Design review of the part built by this model. Coordinates are the model's own, in mm. Coordinates: 2 decimals unless noted, no trailing zeros. Answer as a JSON object with one key per item and string values.
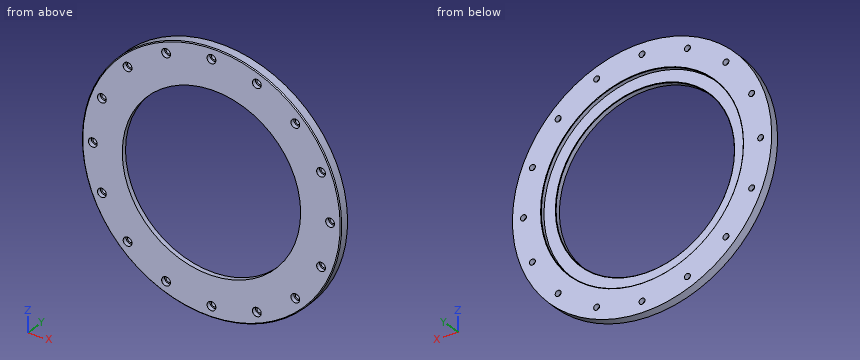
```python
from build123d import *

# Parameters (mm, degrees)
CIRPATTERN1_COUNT = 16
CHAMFER1_SIZE     = 1
CHAMFER2_SIZE     = 2


with BuildPart() as part:
    # Sketch1 → Revolve1 (revolve)
    with BuildSketch(Plane.XY, mode=Mode.PRIVATE) as revolve1_sk:
        Polygon((-203, 0), (-295, 0), (-295, 22), (-230, 22), (-230, 12), (-203, 12), align=None)
    revolve(revolve1_sk.sketch.rotate(Axis((0, 0, 0), (0, 1, 0)), 270), axis=Axis((0, 0, 0), (0, 1, 0)))

    # Sketch4 → CBORE for M12 SHCS1 (revolve, cut)
    with BuildSketch(Plane(origin=(0, 0, 270), x_dir=(0, 0, -1), z_dir=(1, 0, 0))):
        Polygon((0, 0), (0, 22), (6.75, 22), (6.75, 10), (10, 10), (10, 0.025), (10.025, 0), align=None)
    cbore_for_m12_shcs1 = revolve(axis=Axis((0, -6.35, 270), (0, 1, 0)), mode=Mode.SUBTRACT)

    # CirPattern1: CBORE for M12 SHCS1 ×16 about axis
    cirpattern1_axis = Axis((0, 0, 0), (0, 1, 0))
    for i in range(1, CIRPATTERN1_COUNT):
        add(cbore_for_m12_shcs1.rotate(cirpattern1_axis, i * 360 / CIRPATTERN1_COUNT), mode=Mode.SUBTRACT)

    # Chamfer1
    chamfer1_edges = [part.edges().sort_by_distance(p)[0] for p in [
        (0, 12, 203),
        (0, 22, 230),
    ]]
    chamfer(chamfer1_edges, length=CHAMFER1_SIZE)

    # Chamfer2
    chamfer2_edges = [part.edges().sort_by_distance(p)[0] for p in [
        (0, 0, 295),
    ]]
    chamfer(chamfer2_edges, length=CHAMFER2_SIZE)


solid = part.part
```
1) Wall thickness on probe 1 along Z at (x, y) = (-8, 15.5); probe 2 along X at (y, z) = (10.25, -186); probe 3 along Z at (x, y) = (-185, 17.5): over which ranges is each line inside the solid? List them lowest first.
Completed:
{"probe 1": "-294.89 to -229.86, 229.86 to 294.89", "probe 2": "-228.97 to -195.54, -186.3 to -81.32, 81.32 to 186.3, 195.54 to 228.97", "probe 3": "-229.78 to -194.16, -187.67 to -136.66, 136.66 to 187.67, 194.16 to 229.78"}
2) Clearance check with flat-ended pins moving along their axes: pin 1 Ø8 at (y, z) = (10, -186) entering from -X; pin 2 Ø10 at (x, y) = (-123, 17) entering from -Z; pin 3 Ø1.5 at (y, z) = (19.5, -180.5) entering from -X; pin 4 Ø11 at (x, z) = (-190.92, 190.92) entering from +Y. State where each tip first meets the part, or that it passes through.
Completed:
{"pin 1": "x = -232.17", "pin 2": "z = -270.37", "pin 3": "x = -233.91", "pin 4": "through"}
3) Add section A-A, the plane z = 0. Count the separate pieces of the cut face and the enclosed holes in it, and give its area (3 significant figures).
Completed:
{"separate pieces": "4", "enclosed holes": "0", "area": "2,780 mm²"}
